```python
from build123d import *

# Parameters (mm, degrees)
F0_R     = 12.7
F1_DEPTH = 7.1882
F2_R     = 10.795
F3_DEPTH = 4.4831
F4_R     = 6
F5_DEPTH = 25.4
F6_SCALE = 0.5


with BuildPart() as f1:
    # F0 (on Top) → F1 (new body)
    with BuildSketch(Plane.XY):
        Circle(F0_R)
    extrude(amount=F1_DEPTH)

    # F2 (on face) → F3 (join)
    with BuildSketch(Plane.XY):
        Circle(F2_R)
    extrude(amount=-F3_DEPTH)

    # F4 (on face) → F5 (cut)
    with BuildSketch(Plane(origin=(0, 0, -4.4831), x_dir=(1, 0, 0), z_dir=(0, 0, -1))):
        Circle(F4_R)
    extrude(amount=-F5_DEPTH, mode=Mode.SUBTRACT)


with BuildPart() as f1_1:
    # F6: moved
    add(f1.part.scale(F6_SCALE))


solid = f1_1.part
```
CAD build for the part. Positions are in the model's coordinates, mm. A direction names the side the tool comes from. Coordinates: 2 decimals unless noted, no trailing zeros. Write each loop counter-clockwise with the first axis right and the second up, starting at its lowest first coordinate (ties: lowest second). Pieces come first, ordered by that corner, then holes.
(1) 3-axis set-ups, long thin cutter, end or side, ignore diameter. For faces 1 (the face through (2.3, -2.3, -2.242)), 2 (the face through (-3, -5, 0)): which of +Z, -Z, +X, -X, +Y, -Y reach the whole face in a straight line?
(2) Cut at A-A, the plane x = 0. List the corners of the cut face in (y, z), and give its area (3 significant figures).
(3) Drill centre lines: probe 1 along Y at (x, z) = (0, -1); probe 2 along Y at (x, z) = (0, 0.6); probe 3 along X at (y, z) = (-1.75, 2.4). Where is each one in solid material? Low to high.
(4) Cut at D-D, the plane x = -5. List the corners of the cut face in (y, z).
(5) Flat gauge pin, fed straight in: pin 1 (1.5 mm diameter, centred on y = 4, z = 1, fed in from -X). Where does the tip first touch, or does it go through?
(6) Cut at C-C, the plane z = 2.1. List the corners of the cut face in (x, y), and give its area (3 significant figures).
(7) Two-plate mould, pull along X, no slides. Class faces 3 (the face through (-3, 0, 1)), 4 (the face through (3, -1, 3.594)), 5 (the face through (-1.38, -6.2, 1.77)): +X half, -X half, draft (parallel to the pull), parting line (faces both ways), or undercut.
Geometry says:
1. face 1: -Z, +X, -X, +Y, -Y
1. face 2: -Z
2. outline: (-6.35, 0) - (-5.4, 0) - (-5.4, -2.24) - (-3, -2.24) - (-3, 3.59) - (-6.35, 3.59) - close; (3, -2.24) - (5.4, -2.24) - (5.4, 0) - (6.35, 0) - (6.35, 3.59) - (3, 3.59) - close
2. area: 34.8 mm2
3. probe 1: y = -5.4 to -3, 3 to 5.4
3. probe 2: y = -6.35 to -3, 3 to 6.35
3. probe 3: x = -6.1 to -2.44, 2.44 to 6.1
4. outline: (-3.91, 0) - (-2.03, 0) - (-2.03, -2.24) - (2.03, -2.24) - (2.03, 0) - (3.91, 0) - (3.91, 3.59) - (-3.91, 3.59) - close
5. pin 1: stops at x = -5.46
6. outline: circle Ø12.7 at (0, 0); hole circle Ø6 at (0, 0)
6. area: 98.4 mm2
7. face 3: undercut
7. face 4: draft
7. face 5: parting line
